```python
from build123d import *

# Parameters (mm, degrees)
EXTRUDE_1_DEPTH     = 30
EXTRUDE_2_DEPTH     = 3
EXTRUDE_START       = 10
EXTRUDE_3_DEPTH     = 10
SKETCH_4_R          = 1.5
CUT_EXTRUDE_1_DEPTH = 78.719045441
CUT_EXTRUDE_2_DEPTH = 78.27677545
CUT_EXTRUDE_START   = -2.5
CUT_EXTRUDE_3_DEPTH = 81.219045441
FILLET_1_R          = 2


with BuildPart() as part:
    # 草图1 → 凸台-拉伸1 (new body)
    with BuildSketch(Plane.XY):
        with BuildLine():
            Line((-25, -1.5), (25, -1.5))
            ThreePointArc((25, -1.5), (26.5, 0), (25, 1.5))
            Line((25, 1.5), (-25, 1.5))
            add(Edge.make_bspline(
                [(-25, 1.5), (-34.841235479, 1.511543442), (-49.008834865, -3.48233027), (-61.504493466, -11.820085551), (-67.4, -19.7)],
                knots=[0, 0, 0, 0.375, 0.625, 1, 1, 1], degree=2))
            ThreePointArc((-67.4, -19.7), (-67.1, -21.8), (-65, -21.5))
            add(Edge.make_bspline(
                [(-25, -1.5), (-50, -1.5), (-65, -21.5)],
                knots=[0, 0, 0, 1, 1, 1], degree=2))
        make_face()
    extrude(amount=EXTRUDE_1_DEPTH)

    # 草图2 → 凸台-拉伸2 (add)
    with BuildSketch(Plane(origin=(0, 0, 0), x_dir=(-1, 0, 0), z_dir=(0, 0, -1))):
        with BuildLine():
            Line((25, 1.5), (-25, 1.5))
            ThreePointArc((-25, 1.5), (-26.060660172, 1.060660172), (-26.5, 0))
            Line((-26.5, 0), (-26.5, -22.1))
            Line((-26.5, -22.1), (66.2, -22.1))
            ThreePointArc((66.2, -22.1), (67.541640786, -21.270820393), (67.4, -19.7))
            add(Edge.make_bspline(
                [(25, 1.5), (34.841235479, 1.511543442), (49.008834865, -3.48233027), (61.504493466, -11.820085551), (67.4, -19.7)],
                knots=[0, 0, 0, 0.375, 0.625, 1, 1, 1], degree=2))
        make_face()
    extrude(amount=-EXTRUDE_2_DEPTH)

    # 草图3 → 凸台-拉伸3 (add)
    with BuildSketch(Plane(origin=(0, 0, 0), x_dir=(-1, 0, 0), z_dir=(0, 0, -1)).offset(EXTRUDE_START)):
        with BuildLine():
            Line((-25, 1.5), (25, 1.5))
            ThreePointArc((25, 1.5), (26.060660172, 1.060660172), (26.5, 0))
            Line((26.5, 0), (26.5, -5))
            ThreePointArc((26.5, -5), (26.060660172, -6.060660172), (25, -6.5))
            Line((25, -6.5), (-25, -6.5))
            ThreePointArc((-25, -6.5), (-26.060660172, -6.060660172), (-26.5, -5))
            Line((-26.5, -5), (-26.5, 0))
            ThreePointArc((-26.5, 0), (-26.060660172, 1.060660172), (-25, 1.5))
        make_face()
    extrude(amount=-EXTRUDE_3_DEPTH)

    # 草图4 → 切除-拉伸1 (cut, through all)
    with BuildSketch(Plane(origin=(0, 1.5, 0), x_dir=(1, 0, 0), z_dir=(0, 1, 0))):
        with Locations(Location((-13.5, 5, 0), (0, 0, 270))):
            Circle(SKETCH_4_R)
        with Locations(Location((16.5, 5, 0), (0, 0, 270))):
            Circle(SKETCH_4_R)
    extrude(amount=-CUT_EXTRUDE_1_DEPTH, mode=Mode.SUBTRACT)

    # 草图5 → 切除-拉伸2 (cut, through all)
    with BuildSketch(Plane(origin=(0, 0, 0), x_dir=(-1, 0, 0), z_dir=(0, 0, -1))):
        with BuildLine():
            Line((-26.5, -14.5), (33.5, -14.5))
            ThreePointArc((33.5, -14.5), (38.874011537, -16.725988463), (41.1, -22.1))
            Line((41.1, -22.1), (-26.5, -22.1))
            Line((-26.5, -22.1), (-26.5, -14.5))
        make_face()
    extrude(amount=-CUT_EXTRUDE_2_DEPTH, mode=Mode.SUBTRACT)

    # 草图6 → 切除-拉伸3 (cut, through all)
    with BuildSketch(Plane(origin=(0, 1.5, 0), x_dir=(1, 0, 0), z_dir=(0, 1, 0)).offset(CUT_EXTRUDE_START)):
        Polygon((-11.91228676, 7.75), (-15.08771324, 7.75), (-16.675426481, 5), (-15.08771324, 2.25), (-11.91228676, 2.25), (-10.324573519, 5), align=None)
        Polygon((18.08771324, 7.75), (14.91228676, 7.75), (13.324573519, 5), (14.91228676, 2.25), (18.08771324, 2.25), (19.675426481, 5), align=None)
    extrude(amount=CUT_EXTRUDE_3_DEPTH, mode=Mode.SUBTRACT)

    # 圆角1
    fillet_1_edges = [part.edges().sort_by_distance(p)[0] for p in [
        (-41.1, -22.1, 1.5),
    ]]
    fillet(fillet_1_edges, radius=FILLET_1_R)


solid = part.part
```
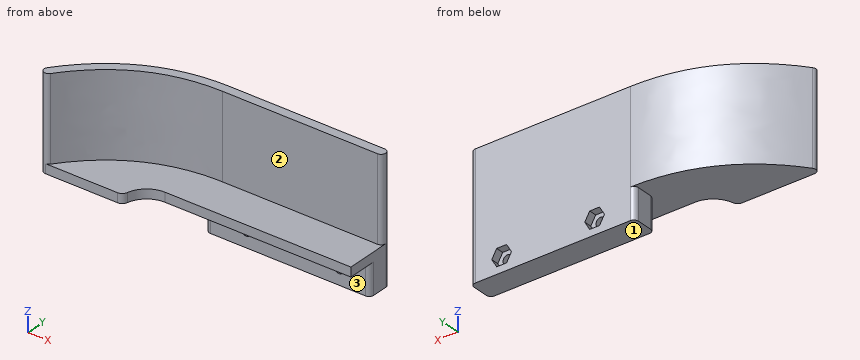
Here's how the part is built. I have some questions about the finished solid (model axes, mm). Face numbers are marked on the shaded views. A direction names the side the tool comes from. Coordinates: 2 decimals unless noted, no trailing zeros. Loops run counter-clockwise (first coordinate to the right, second up) from the corner with the lowest first, then second, coordinate; pieces in that order, holes last. Notation, with made-up numbers: M -35.75,81.25 L -22.75,81.25 A30 cw -22.75,106.25 Z; hole C 2.5,15 d6. An arc over 180 degrees is marked long. One line per item, written item: value.
1. Will these pins go through, and if not, where does the flat tip stop? pin 1 Ø5.5 at (y, z) = (-2.5, -4.5) entering from -X; pin 2 Ø2 at (y, z) = (-12, 13.5) entering from -X; pin 3 Ø6 at (x, z) = (15, -4) entering from +Y; pin 4 Ø8 at (x, z) = (-20.5, 7.5) entering from -Y.
Geometry says:
pin 1: stops at x = -26.5
pin 2: stops at x = -61.58
pin 3: stops at y = 1.5
pin 4: stops at y = -1.5
2. Imagine slicing it at A-A (x = -13.5). List the corners of the cut face in (y, z) for me.
Geometry says:
outline: M -14.5,0 L -6.5,0 L -6.5,-3.5 L -1,-3.5 L -1,-2.25 L 1.5,-2.25 L 1.5,30 L -1.5,30 L -1.5,3 L -14.5,3 Z; M -6.5,-10 L 1.5,-10 L 1.5,-7.75 L -1,-7.75 L -1,-6.5 L -6.5,-6.5 Z
3. Please list where these lines run through material, in increasing order: probe 1 along X at (y, z) = (-3.55, -5); probe 2 along Y at (x, z) = (-25.5, 15.5); probe 3 along Z at (x, y) = (21, -2.25).
Geometry says:
probe 1: x = -26.5 to -15, -12 to 15, 18 to 26.5
probe 2: y = -1.5 to 1.5
probe 3: z = -10 to 3
4. Imagine slicing it at B-B (x = 7). List the corners of the cut face in (y, z) for me, and give its area (3 significant figures).
Geometry says:
outline: M -14.5,0 L -6.5,0 L -6.5,-10 L 1.5,-10 L 1.5,30 L -1.5,30 L -1.5,3 L -14.5,3 Z
area: 209 mm2
5. On a 3-axis mill with a long thin cutter (end or side, diameter ignored), from which of +Z, -Z, +X, -X, +Y, -Y can I reach the whole of each face in a straight line? I mean the marked faces 1, 2 and 3. Say none if no direction works.
Geometry says:
face 1: -Z, +X, -X, +Y, -Y
face 2: +Z, +X, -Y
face 3: -Z, +X, -X, -Y
